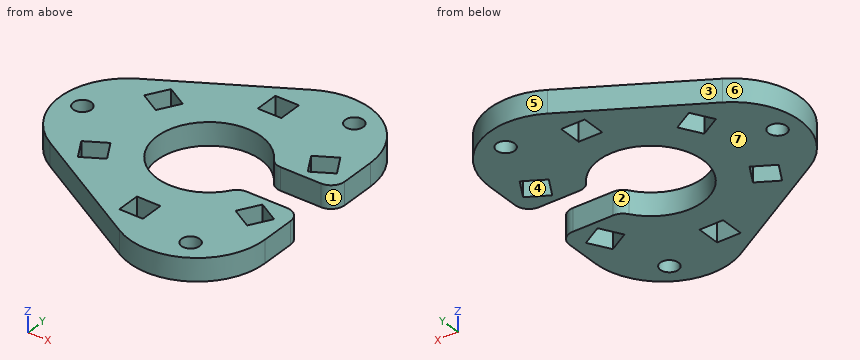
from build123d import *

# Parameters (mm, degrees)
SKETCH1_R           = 2
SKETCH1_W           = 5.2
SKETCH1_H           = 5.2
BOSS_EXTRUDE1_DEPTH = 5
CONG_1_R            = 15
CONG_2_R            = 3


with BuildPart() as part:
    # Sketch1 → Boss-Extrude1 (new body)
    with BuildSketch(Plane.XY):
        with BuildLine():
            Line((24, 5), (24, 41.569219382))
            Line((24, 41.569219382), (-48, 0))
            Line((-48, 0), (24, -41.569219382))
            Line((24, -41.569219382), (24, -5))
            Line((24, -5), (10.356157589, -5))
            ThreePointArc((10.356157589, -5), (-11.5, 0), (10.356157589, 5))
            Line((10.356157589, 5), (24, 5))
        make_face()
        with Locations((14, 24.248711306)):
            Circle(SKETCH1_R, mode=Mode.SUBTRACT)
        with Locations((14, -24.248711306)):
            Circle(SKETCH1_R, mode=Mode.SUBTRACT)
        with Locations((-28, 0)):
            Circle(SKETCH1_R, mode=Mode.SUBTRACT)
        with Locations((0, 20.5)):
            Rectangle(SKETCH1_W, SKETCH1_H, mode=Mode.SUBTRACT)
        Polygon((21.305186827, 9.29833395), (16.801854728, 6.69833395), (14.201854728, 11.20166605), (18.705186827, 13.80166605), align=None, mode=Mode.SUBTRACT)
        Polygon((18.705186827, -13.80166605), (14.201854728, -11.20166605), (16.801854728, -6.69833395), (21.305186827, -9.29833395), align=None, mode=Mode.SUBTRACT)
        with Locations((0, -20.5)):
            Rectangle(SKETCH1_W, SKETCH1_H, mode=Mode.SUBTRACT)
        Polygon((-21.305186827, -9.29833395), (-16.801854728, -6.69833395), (-14.201854728, -11.20166605), (-18.705186827, -13.80166605), align=None, mode=Mode.SUBTRACT)
        Polygon((-18.705186827, 13.80166605), (-14.201854728, 11.20166605), (-16.801854728, 6.69833395), (-21.305186827, 9.29833395), align=None, mode=Mode.SUBTRACT)
    extrude(amount=BOSS_EXTRUDE1_DEPTH)

    # Congé1
    cong_1_edges = [part.edges().sort_by_distance(p)[0] for p in [
        (24, -41.569219382, 2.5),
        (-48, 0, 2.5),
        (24, 41.569219382, 2.5),
    ]]
    fillet(cong_1_edges, radius=CONG_1_R)

    # Congé2
    cong_2_edges = [part.edges().sort_by_distance(p)[0] for p in [
        (10.356157589, 5, 2.5),
        (10.356157589, -5, 2.5),
        (24, -5, 2.5),
        (24, 5, 2.5),
    ]]
    fillet(cong_2_edges, radius=CONG_2_R)


solid = part.part
For this review, take the finished solid that the model builds, in its own axes (mm). Face numbers are marked on the shaded views. A direction names the side the tool comes from. Coordinates: 2 decimals unless noted, no trailing zeros. Order: outer loops, then holes, each group sorted by start corner. A loop starts at its lowest first (then second) coordinate and runs counter-clockwise, first axis right, second up. Notation, with made-up numbers: (-35, -7) - (-29, -7) arc R18 ccw to (-29, 14) - close; hole circle Ø4 at (58.5, 2). An arc over 180 degrees is marked (long way). Use one line per item in the form item = value.
Q1. Consider section A-A (y = 0). Give the boundary of the cut face in (x, z).
Checked values:
outline = (-33, 0) - (-30, 0) - (-30, 5) - (-33, 5) - close; (-26, 0) - (-11.5, 0) - (-11.5, 5) - (-26, 5) - close
Q2. Consider section D-D (z = 2.5). Give the number of separate pieces and of enclosed holes in the cut face, then the cut area to 3 significant figures.
Checked values:
separate_pieces = 1
enclosed_holes = 9
area = 1,780 mm2
Q3. Draft analysis for pull direction Y (two halves, no side actions). For the marked faces 4, 5, 6 and 7, state which applies: +Y half, -Y half, draft (parallel to the pull), parting line (faces both ways), or undercut.
Checked values:
face_4 = undercut
face_5 = +Y half
face_6 = parting line
face_7 = draft
Q4. For the marked faces 1, 2 and 3, list the 3-axis set-ups (+Z, -Z, +X, -X, +Y, -Y) from which the entire face can be reached by the end or side of a thin tool; tool diameter is ignored.
Checked values:
face_1 = +Z, -Z, +X
face_2 = +Z, -Z
face_3 = +Z, -Z, -X, +Y
Q5. Consider section C-C (x = 0). Give the boundary of the cut face in (y, z).
Checked values:
outline = (-27.71, 0) - (-23.1, 0) - (-23.1, 5) - (-27.71, 5) - close; (-17.9, 0) - (-11.5, 0) - (-11.5, 5) - (-17.9, 5) - close; (11.5, 0) - (17.9, 0) - (17.9, 5) - (11.5, 5) - close; (23.1, 0) - (27.71, 0) - (27.71, 5) - (23.1, 5) - close
Q6. For P1, Ø1.5, axis at x = -2.5, z = 2, coming from the +Y side; P2, Ø2.5, axis at x = 0.5, z = 3, coming from the +Y side; P3, Ø3, axis at x = -16, z = 1.5, coming from the -Y side; P4, Ø3.5, axis at x = 14, y = 24.25, coming from the -Z side, all flat-tipped, find the tip position at first contact; note any pin that passes through.
Checked values:
P1 = 26.7
P2 = 28.72
P3 = -19.34
P4 = through
Q7. Consider section B-B (x = -28). Give the boundary of the cut face in (y, z), then the cut area to 3 significant figures.
Checked values:
outline = (-11.18, 0) - (-2, 0) - (-2, 5) - (-11.18, 5) - close; (2, 0) - (11.18, 0) - (11.18, 5) - (2, 5) - close
area = 91.8 mm2
Q8. For probe 1 along X at (y, z) = (-13, 1.5); probe 2 along Y at (x, z) = (17, 4.55); probe 3 along Y at (x, z) = (-20, 2.5), list the stretches that pass through material, from the lowest coordinate up. Write a range as from..to.
Checked values:
probe_1 = -25.48..-19.17, -17.32..17.32, 19.17..24
probe_2 = -28.28..-12.82, -6.81..-5, 5..6.81, 12.82..28.28
probe_3 = -16.17..-11.56, -8.54..8.54, 11.56..16.17
